The listing builds one solid part. Answer for the finished solid, in the listing's coordinates (mm). A direction names the side the tool comes from. Round coordinates to 2 decimals unless told otherwise and drop trailing zeros. Loops run counter-clockwise (first coordinate to the right, second up) from the corner with the lowest first, then second, coordinate; pieces in that order, holes last. Notation, with made-up numbers: (-40, 28.5) -> (-2, 28.5) arc R37 cw to (-2, 65.5) -> close; hole circle Ø6 at (3.5, 72.25). An arc over 180 degrees is marked (long way). Use a Markdown table: item, result. Add a question column.
Q1. Section C-C on x = 12.5 is taken. Give the vertices of the cut face in (y, z).
Q2. Given pin 1 Ø1 at (y, z) = (-5, -14) entering from -X; pin 2 Ø8 at (x, z) = (22, -35.5) entering from -Y; pin 3 Ø10.5 at (x, z) = (15, -16) entering from +Y, each flat-ended and moving along its own axis, determine where each tip first touches the part or whether it passes through.
Q3. Section D-D on z = -35.5 is taken. Give the vertices of the cut face in (x, y), then the cut area to 3 significant figures.
Q4. For a pull along X with two mould halves and no side action, classify faces 1 (the flat face through (25, 5, -21)), 2 (the flat face through (12, 2, -20)), 3 (the flat face through (12.3, 1.5, 0)) as released by +X, released by -X, zero draft, split by the parting line, or undercut.
Q5. Which of the six approach directions +Z, -Z, +X, -X, +Y, -Y give full straight-line access (tool end or side, diameter ignored) to faces 4 (the flat face through (13, 5, -42)), 5 (the cylindrical face through (14.9, -4.9, -13.2)), 6 (the flat face through (13, 6, -40))?
Q6. Consider line 1 (X direction, y = 5, z = -34); line 2 (Y direction, x = 24, z = -24); line 3 (Z direction, x = 20, y = 8.25). Determine where each line is inside the solid, lowest interval first.
Q7. Section B-B on z = -10 is taken. Give the vertices of the cut face in (x, y), then the cut area to 3 significant figures.
Q8. Section A-A on y = 6.5 is taken. Give the vertices of the cut face in (x, z), then the cut area to 3 significant figures.
from build123d import *

# Parameters (mm, degrees)
SKETCH1_W           = 25
SKETCH1_H           = 40
BOSS_EXTRUDE1_DEPTH = 2
SKETCH2_W           = 2
SKETCH2_H           = 40
BOSS_EXTRUDE2_DEPTH = 7.5
SKETCH3_R           = 4
BOSS_EXTRUDE3_DEPTH = 10
SKETCH4_W           = 25
SKETCH4_H           = 9.5
BOSS_EXTRUDE4_DEPTH = 2


with BuildPart() as part:
    # Sketch1 → Boss-Extrude1 (new body)
    with BuildSketch(Plane(origin=(0, 0, 0), x_dir=(1, 0, 0), z_dir=(0, 1, 0))):
        with Locations((12.5, 20)):
            Rectangle(SKETCH1_W, SKETCH1_H)
    extrude(amount=BOSS_EXTRUDE1_DEPTH)

    # Sketch2 → Boss-Extrude2 (add)
    with BuildSketch(Plane(origin=(0, 2, 0), x_dir=(1, 0, 0), z_dir=(0, 1, 0))):
        with Locations((1, 20)):
            Rectangle(SKETCH2_W, SKETCH2_H)
        with Locations((24, 20)):
            Rectangle(SKETCH2_W, SKETCH2_H)
    extrude(amount=BOSS_EXTRUDE2_DEPTH)

    # Sketch3 → Boss-Extrude3 (add)
    with BuildSketch(Plane(origin=(0, 0, 0), x_dir=(-1, 0, 0), z_dir=(0, -1, 0))):
        with Locations(Location((-12.5, 10, 0), (0, 0, 270))):
            Circle(SKETCH3_R)
    extrude(amount=BOSS_EXTRUDE3_DEPTH)

    # Sketch4 → Boss-Extrude4 (add)
    with BuildSketch(Plane(origin=(0, 0, -40), x_dir=(-1, 0, 0), z_dir=(0, 0, -1))):
        with Locations((-12.5, 4.75)):
            Rectangle(SKETCH4_W, SKETCH4_H)
    extrude(amount=BOSS_EXTRUDE4_DEPTH)


solid = part.part
Checked values:
| question | item | result |
|---|---|---|
| 1 | outline | (-10, -14) -> (0, -14) -> (0, -42) -> (9.5, -42) -> (9.5, -40) -> (2, -40) -> (2, 0) -> (0, 0) -> (0, -6) -> (-10, -6) -> close |
| 2 | pin 1 | stops at x = 10.56 |
| 2 | pin 2 | stops at y = 0 |
| 2 | pin 3 | stops at y = 2 |
| 3 | outline | (0, 0) -> (25, 0) -> (25, 9.5) -> (23, 9.5) -> (23, 2) -> (2, 2) -> (2, 9.5) -> (0, 9.5) -> close |
| 3 | area | 80.0 mm2 |
| 4 | face 1 | released by +X |
| 4 | face 2 | undercut |
| 4 | face 3 | zero draft |
| 5 | face 4 | -Z, +X, -X, +Y, -Y |
| 5 | face 5 | -Y |
| 5 | face 6 | +Z, +Y |
| 6 | line 1 | x = 0 to 2, 23 to 25 |
| 6 | line 2 | y = 0 to 9.5 |
| 6 | line 3 | z = -42 to -40 |
| 7 | outline | (0, 0) -> (8.5, 0) -> (8.5, -10) -> (16.5, -10) -> (16.5, 0) -> (25, 0) -> (25, 9.5) -> (23, 9.5) -> (23, 2) -> (2, 2) -> (2, 9.5) -> (0, 9.5) -> close |
| 7 | area | 160 mm2 |
| 8 | outline | (0, -42) -> (25, -42) -> (25, 0) -> (23, 0) -> (23, -40) -> (2, -40) -> (2, 0) -> (0, 0) -> close |
| 8 | area | 210 mm2 |
